```python
from build123d import *

# Parameters (mm, degrees)
FILLET1_R  = 1.5
SKETCH2_W  = 11.3
SKETCH2_H  = 1.6
SLOT_DEPTH = 1.6


with BuildPart() as part:
    # BodySke → Base-Revolve (revolve)
    with BuildSketch(Plane.XY, mode=Mode.PRIVATE) as base_revolve_sk:
        Polygon((0, 0), (0, 5.65), (0.65, 5.65), (3.3, 3), (10, 3), (10, 0), align=None)
    revolve(base_revolve_sk.sketch.rotate(Axis((-6.35, 0, 0), (1, 0, 0)), 90), axis=Axis((-6.35, 0, 0), (1, 0, 0)))  # turned: the seam where the file's is

    # Fillet1
    fillet1_edges = [part.edges().sort_by_distance(p)[0] for p in [
        (3.3, 0, -3),
    ]]
    fillet(fillet1_edges, radius=FILLET1_R)

    # Sketch2 → Slot (cut)
    with BuildSketch(Plane.ZY):
        Rectangle(SKETCH2_W, SKETCH2_H)
    extrude(amount=-SLOT_DEPTH, mode=Mode.SUBTRACT)


solid = part.part
```
Model file for the job. Use its own axes, mm. A direction names the side the tool comes from. Round coordinates to 2 decimals unless told otherwise and drop trailing zeros. Write each loop counter-clockwise with the first axis right and the second up, starting at its lowest first coordinate (ties: lowest second). Pieces come first, ordered by that corner, then holes. Notation, with made-up numbers: (24, 79.5) -> (46, 79.5) arc R19 cw to (46, 113.5) -> close; hole circle Ø4 at (46.5, 67.25). An arc over 180 degrees is marked (long way). Answer as CSV lines item,"result".
1. Drill centre lines: line 1 (Y direction, x = 1, z = 2.5); line 2 (Z direction, x = 3.5, y = 2.25); line 3 (Y direction, x = 5, z = -1.25). Where is each one in solid material? Low to high.
Resolved:
line 1,"-4.67 to -0.8, 0.8 to 4.67"
line 2,"-2.07 to 2.07"
line 3,"-2.73 to 2.73"
2. Tool access for faces 4 (the face through (0, -3, 0)), 5 (the face through (1.6, 0, 0)), 6 (the face through (7, -0.9, 2.86)): list every direction of +Z, -Z, +X, -X, +Y, -Y with a clear straight run to the whole face (end or side of a thin tool).
Resolved:
face 4,"+Z, -Z, -X, +Y, -Y"
face 5,"+Z, -Z, -X"
face 6,"+X"
3. Slice it at A-A, the plane x = 8.25. List the corners of the cut face in (y, z), plus the area to 3 significant figures.
Resolved:
outline,"circle Ø6 at (0, 0)"
area,"28.3 mm²"
4. Pin check, flat tips, straight feed: pin 1 Ø3 at (x, z) = (4.5, 3) entering from +Y; pin 2 Ø0.5 at (x, z) = (1, 1.5) entering from -Y; pin 3 Ø5 at (x, y) = (8, 4) entering from -Z. Stop position of each tip, or through.
Resolved:
pin 1,"y = 2.6"
pin 2,"y = -5.35"
pin 3,"z = -2.6"
5. Mould opens along Y. For faces 1 (the face through (1, 0.8, 0)), 2 (the face through (0, 3, 0)), 3 (the face through (0.33, 5.65, -0.11)) say: +Y half, -Y half, draft (parallel to the pull), parting line (faces both ways), or undercut.
Resolved:
face 1,"undercut"
face 2,"draft"
face 3,"+Y half"
